Read the model definition and answer for the solid it produces. Units are mm, in the model's axes. Coordinates: 2 decimals unless noted, no trailing zeros. Order: outer loops, then holes, each group sorted by start corner. A loop starts at its lowest first (then second) coordinate and runs counter-clockwise, first axis right, second up. Notation, with made-up numbers: (47.5, 37) -> (61.5, 37) arc R25 cw to (61.5, 69) -> close; hole circle Ø7 at (85.5, 49.5). An arc over 180 degrees is marked (long way). Return JSON: item names as keys, results as strings. Group by question number.
```python
from build123d import *

# Parameters (mm, degrees)
SKETCH1_W           = 26
SKETCH1_H           = 12
BOSS_EXTRUDE1_DEPTH = 1.5
SKETCH2_R           = 2.25
CUT_EXTRUDE1_DEPTH  = 2.5


with BuildPart() as part:
    # Sketch1 → Boss-Extrude1 (new body)
    with BuildSketch(Plane(origin=(0, 0, 0), x_dir=(1, 0, 0), z_dir=(0, 1, 0))):
        Rectangle(SKETCH1_W, SKETCH1_H)
    extrude(amount=BOSS_EXTRUDE1_DEPTH)

    # Sketch2 → Cut-Extrude1 (cut, through all)
    with BuildSketch(Plane(origin=(0, 1.5, 0), x_dir=(1, 0, 0), z_dir=(0, 1, 0))):
        with Locations(Location((-6.25, 0, 0), (0, 0, 270))):  # turned: the seam where the file's is
            Circle(SKETCH2_R)
    cut_extrude1 = extrude(amount=-CUT_EXTRUDE1_DEPTH, mode=Mode.SUBTRACT)

    # Mirror1: Cut-Extrude1 across plane
    add(cut_extrude1.mirror(Plane(origin=(0, 0, 0), x_dir=(0, 0, 1), z_dir=(1, 0, 0))), mode=Mode.SUBTRACT)


solid = part.part
```
1. Given pin 1 (2.5 mm diameter, centred on x = 6.25, z = 0, fed in from +Y), flat-ended and moving along its own axis, determine where the tip first touches the part or whether it passes through.
2. Find section A-A on z = 0. Determine the outline of the cut face in (x, y).
3. Find section B-B on x = -6.25. Determine the outline of the cut face in (y, z), and give its area (4 significant figures).
4. Find section C-C on y = 0.5. Determine the outline of the cut face in (x, z).
5. For a pull along Z with two mould halves and no side action, classify faces 1 (the face through (-4, 1, 0)), 2 (the face through (0, 1, -6)), 3 (the face through (-13, 1, 0)) as released by +Z, released by -Z, zero draft, split by the parting line, or undercut.
6. Straight lines are drawn through the part: L1, parallel to X at y = 1.2, z = 0; L2, parallel to X at y = 0.6, z = 0.75; L3, parallel to Z at x = -5, y = 0.35. For each, find the intervals that lie inside material, in ascending order.
7. Find section D-D on x = 6.5. Determine the outline of the cut face in (y, z).
Result:
{
 "1": {"pin 1": "through"},
 "2": {"outline": "(-13, 0) -> (-8.5, 0) -> (-8.5, 1.5) -> (-13, 1.5) -> close; (-4, 0) -> (4, 0) -> (4, 1.5) -> (-4, 1.5) -> close; (8.5, 0) -> (13, 0) -> (13, 1.5) -> (8.5, 1.5) -> close"},
 "3": {"outline": "(0, -6) -> (1.5, -6) -> (1.5, -2.25) -> (0, -2.25) -> close; (0, 2.25) -> (1.5, 2.25) -> (1.5, 6) -> (0, 6) -> close", "area": "11.25 mm^2"},
 "4": {"outline": "(-13, -6) -> (13, -6) -> (13, 6) -> (-13, 6) -> close; hole circle Ø4.5 at (-6.25, 0); hole circle Ø4.5 at (6.25, 0)"},
 "5": {"face 1": "undercut", "face 2": "released by -Z", "face 3": "zero draft"},
 "6": {"L1": "-13 to -8.5, -4 to 4, 8.5 to 13", "L2": "-13 to -8.37, -4.13 to 4.13, 8.37 to 13", "L3": "-6 to -1.87, 1.87 to 6"},
 "7": {"outline": "(0, -6) -> (1.5, -6) -> (1.5, -2.24) -> (0, -2.24) -> close; (0, 2.24) -> (1.5, 2.24) -> (1.5, 6) -> (0, 6) -> close"}
}
